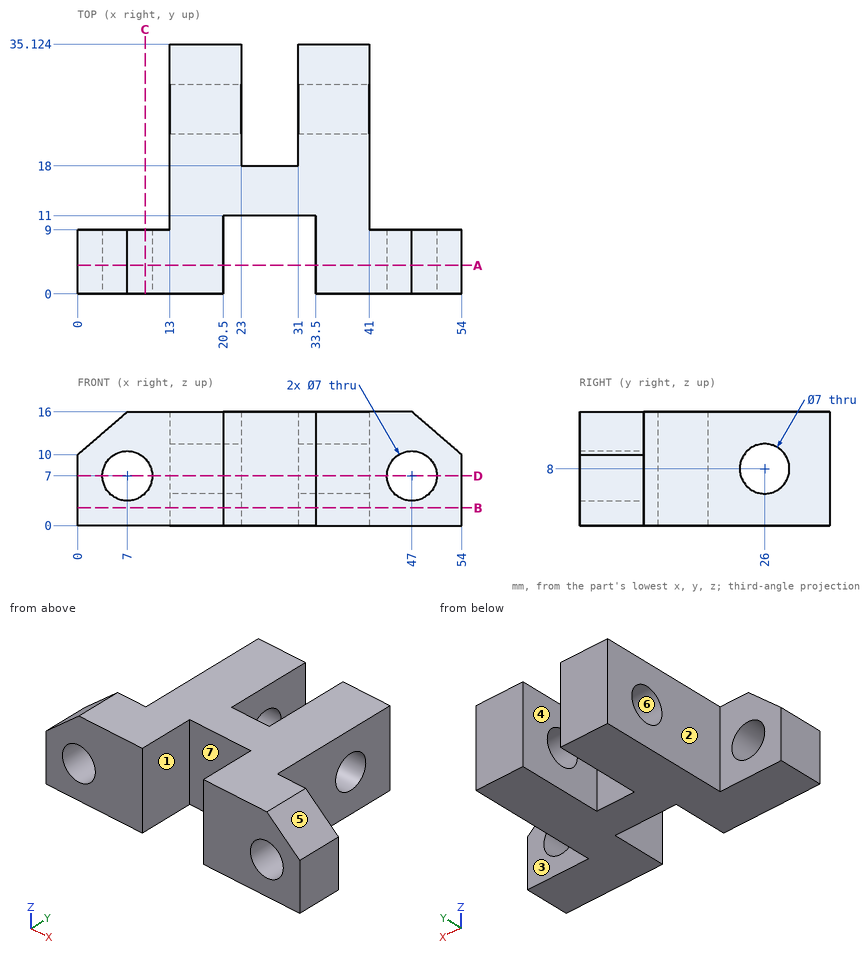
The figure shows three views and two pictorial views of one solid part (mm, origin at its lowest corner). Answer the questions. A direction names the side the tool comes from. Give positions to 0.01 mm unless a question says otherwise; leave off trailing zeros. Order: outer loops, then holes, each group sorted by start corner. A loop starts at its lowest first (then second) coordinate and runs counter-clockwise, first axis right, second up. Notation, with made-up numbers: (56, 8.25) -> (83, 8.25) arc R9 ccw to (83, 17.25) -> close; hole circle Ø3 at (60, 84). An arc over 180 degrees is marked (long way). Answer as CSV lines item,"result". Start each with the question number.
(1) Section A-A, the plane y = 4 is taken. Write down the section's boundary in (x, z).
(2) Which of the six approach directions +Z, -Z, +X, -X, +Y, -Y give full straight-line access (tool end or side, diameter ignored) to the marked faces 1, 2, 3 and 4?
(3) For a pull along Z with two mould halves and no side action, classify the marked faces 5, 6 and 7 as released by +Z, released by -Z, zero draft, split by the parting line, or undercut.
(4) Each of these flat-tipped pins is pushed along its axis until it touches: pin 1 Ø4 at (x, z) = (45, 8.5) entering from +Y; pin 2 Ø9 at (y, z) = (26, 8) entering from -X; pin 3 Ø6.5 at (x, z) = (26.5, 10.5) entering from -Y. Where does it stop, or does it pass through?
(5) Section D-D, the plane z = 7 is taken. Give the number of separate pieces and of enclosed holes in the cut face, plus the area to 3 significant figures.
(6) Section B-B, the plane z = 2.5 is taken. Write down the section's boundary in (x, y).
(7) Consider line 1 along X through (y, z) = (4.75, 7); line 2 along Y through (x, z) = (17.5, 8); line 3 along X through (y, z) = (6, 6). Determine where each line is inside the solid, lowest interval first.
(8) Section C-C, the plane x = 9.5 is taken. Write down the section's boundary in (y, z).
Entries:
1,outline,"(0, 0) -> (20.5, 0) -> (20.5, 16) -> (7, 16) -> (0, 10) -> close; (33.5, 0) -> (54, 0) -> (54, 10) -> (47, 16) -> (33.5, 16) -> close; hole circle Ø7 at (7, 7); hole circle Ø7 at (47, 7)"
2,face 1,"+Z, -Z, -Y"
2,face 2,"+Z, -Z, -X, +Y"
2,face 3,"+Z, -Z, +X, +Y"
2,face 4,"+Z, -Z, +Y"
3,face 5,"released by +Z"
3,face 6,"undercut"
3,face 7,"zero draft"
4,pin 1,"y = 9"
4,pin 2,"x = 13"
4,pin 3,"y = 11"
5,separate pieces,"5"
5,enclosed holes,"0"
5,area,"677 mm²"
6,outline,"(0, 0) -> (20.5, 0) -> (20.5, 11) -> (33.5, 11) -> (33.5, 0) -> (54, 0) -> (54, 9) -> (41, 9) -> (41, 35.12) -> (31, 35.12) -> (31, 18) -> (23, 18) -> (23, 35.12) -> (13, 35.12) -> (13, 9) -> (0, 9) -> close"
7,line 1,"0 to 3.5, 10.5 to 20.5, 33.5 to 43.5, 50.5 to 54"
7,line 2,"0 to 22.5, 29.5 to 35.12"
7,line 3,"0 to 3.65, 10.35 to 20.5, 33.5 to 43.65, 50.35 to 54"
8,outline,"(0, 0) -> (9, 0) -> (9, 4.55) -> (0, 4.55) -> close; (0, 9.45) -> (9, 9.45) -> (9, 16) -> (0, 16) -> close"
